Verification items for the finished model (mm, model axes). Give positions to 0.01 mm unless a question says otherwise; leave off trailing zeros. Order: outer loops, then holes, each group sorted by start corner. A loop starts at its lowest first (then second) coordinate and runs counter-clockwise, first axis right, second up.
Autodesk Inventor part; units mm, degrees
ref_plane "Dummy_IR_XY" through (0, 0, 0) normal (1, 0, 0) x (0, 0, -1)
ref_plane "Dummy_IR_YZ" through (0, 0, 0) normal (0, 0, -1) x (0, 1, 0)
ref_plane "Dummy_IR_ZX" through (0, 0, 0) normal (0, 1, 0) x (1, 0, 0)
sketch "Sketch_3" plane through (0, 0, 0) normal (0, 0, 1) x (1, 0, 0)
  line L0 (5, 0) -> (0, 0)
  line L1 (0, 4.25) -> (0.25, 4)
  line L2 (0.25, 4) -> (4.75, 4)
  line L3 (4.75, 4) -> (5, 4.25)
  line L4 (5, 4.25) -> (5, 5.75)
  line L5 (5, 5.75) -> (4.75, 6)
  line L6 (4.75, 6) -> (3.8856, 6)
  arc A0 (1.1144, 6) -> (3.8856, 6) centre (2.5, 6.8) ccw
  line L7 (1.1144, 6) -> (0.25, 6)
  line L8 (0.25, 6) -> (0, 5.75)
  line L9 (0, 5.75) -> (0, 4.25)
revolve "Revolution1" add sketch "Sketch_3" angle 360 about axis through (5, 0, 0) along (1, 0, 0)
ref_plane "Dummy_IR_XY" through (0, 0, 0) normal (1, 0, 0) x (0, 0, -1)
ref_plane "Dummy_IR_YZ" through (0, 0, 0) normal (0, 0, -1) x (0, 1, 0)
ref_plane "Dummy_IR_ZX" through (0, 0, 0) normal (0, 1, 0) x (1, 0, 0)
ref_plane "IR_OR_XY" through (0, 0, 0) normal (1, 0, 0) x (0, 0, -1)
ref_plane "IR_OR_YZ" through (0, 0, 0) normal (0, 0, -1) x (0, 1, 0)
ref_plane "IR_OR_ZX" through (0, 0, 0) normal (0, 1, 0) x (1, 0, 0)
properties part number "040102DR-18-H8_ir_CPY"
(1) Section check C-C, the plane x = 4.4. Enter the section's corners in (y, z), then the cut area to 3 significant figures.
Solved:
outline: circle Ø12 at (0, 0); hole circle Ø8 at (0, 0)
area: 62.8 mm2
(2) Section check D-D, the plane x = 2.7. Enter the section's corners in (y, z), then the cut area to 3 significant figures.
Solved:
outline: circle Ø10.43 at (0, 0); hole circle Ø8 at (0, 0)
area: 35.1 mm2
(3) Scan lines: line 1 (Z direction, x = 4.7, y = 0); line 2 (Z direction, x = 1.65, y = 0); line 3 (X direction, y = 4.5, z = -3). Record each from-to range of solid material in increasing order.
Solved:
line 1: z = -6 to -4, 4 to 6
line 2: z = -5.44 to -4, 4 to 5.44
line 3: x = 0 to 1.71, 3.29 to 5
(4) Go/stop test with flat-tipped pins: pin 1 (2 mm diameter, centred on x = 2, z = 3, fed in from +Y); pin 2 (1.5 mm diameter, centred on x = 3.5, z = 2, fed in from -Y); pin 3 (1 mm diameter, centred on x = 3, z = 2, fed in from +Y). Record where each tip stops, or that it passes through.
Solved:
pin 1: stops at y = 5.44
pin 2: stops at y = -5.84
pin 3: stops at y = 5.22
(5) Section check A-A, the plane z = 0. Enter the section's corners in (x, y), then the cut area to 3 significant figures.
Solved:
outline: (0, -5.75) - (0.25, -6) - (1.11, -6) arc R1.6 cw to (3.89, -6) - (4.75, -6) - (5, -5.75) - (5, -4.25) - (4.75, -4) - (0.25, -4) - (0, -4.25) - close; (0, 4.25) - (0.25, 4) - (4.75, 4) - (5, 4.25) - (5, 5.75) - (4.75, 6) - (3.89, 6) arc R1.6 cw to (1.11, 6) - (0.25, 6) - (0, 5.75) - close
area: 16.6 mm2
(6) Release check for a two-part mould opening along Z. For faces 1 (the cylindrical face through (2.532, -0.867, -3.905)), 2 (the cylindrical face through (0.676, -5.994, -0.264)), 3 (the flat face through (5, -2, -4)) record: pulls with the +Z half, pulls with the -Z half, needs draft (parallel to the pull), parting line crosses it, or undercut.
Solved:
face 1: undercut
face 2: parting line crosses it
face 3: needs draft
